Build history of the part. All positions in model axes, mm. Face numbers are marked on the shaded views. A direction names the side the tool comes from. Round coordinates to 2 decimals unless told otherwise and drop trailing zeros. Write each loop counter-clockwise with the first axis right and the second up, starting at its lowest first coordinate (ties: lowest second). Pieces come first, ordered by that corner, then holes. Notation, with made-up numbers: (43, 35.5) -> (75, 35.5) arc R20 ccw to (75, 44.5) -> close; hole circle Ø6 at (80, 44.25). An arc over 180 degrees is marked (long way). Return JSON: item names as keys, results as strings.
from build123d import *

# Parameters (mm, degrees)
F0_W      = 76.2
F0_H      = 50.8
F0_R      = 12.7
F1_DEPTH  = 19.05
F2_R      = 5.08
F3_R      = 5.08
F4_R      = 5.08
F6_DEPTH  = 2.54
F7_R      = 4.7625
F8_DEPTH  = 19.05
F10_DEPTH = 50.801


with BuildPart() as f1:
    # F0 (on Top) → F1 (new body)
    with BuildSketch(Plane.XY):
        Rectangle(F0_W, F0_H)
        Circle(F0_R, mode=Mode.SUBTRACT)
    extrude(amount=F1_DEPTH)

    # F2
    f2_edges = [f1.edges().sort_by_distance(p)[0] for p in [
        (-38.1, -25.4, 9.525),
    ]]
    fillet(f2_edges, radius=F2_R)

    # F3
    f3_edges = [f1.edges().sort_by_distance(p)[0] for p in [
        (38.1, -25.4, 9.525),
        (38.1, 25.4, 9.525),
    ]]
    fillet(f3_edges, radius=F3_R)

    # F4
    f4_edges = [f1.edges().sort_by_distance(p)[0] for p in [
        (-38.1, 25.4, 9.525),
    ]]
    fillet(f4_edges, radius=F4_R)

    # F5 (on face) → F6 (cut)
    with BuildSketch(Plane.XY.offset(19.05)):
        with BuildLine():
            Line((-29.21, 25.4), (-33.02, 25.4))
            ThreePointArc((-33.02, 25.4), (-34.3348007491, 25.2269031975), (-35.56, 24.7194090512))
            Line((-35.56, 24.7194090512), (-35.56, -24.7194090512))
            ThreePointArc((-35.56, -24.7194090512), (-34.3348007491, -25.2269031975), (-33.02, -25.4))
            Line((-33.02, -25.4), (-29.21, -25.4))
            Line((-29.21, -25.4), (-29.21, 25.4))
        make_face()
        with BuildLine():
            Line((-6.35, -10.9985226281), (-6.35, -25.4))
            Line((-6.35, -25.4), (6.35, -25.4))
            Line((6.35, -25.4), (6.35, -10.9985226281))
            ThreePointArc((6.35, -10.9985226281), (0, -12.7), (-6.35, -10.9985226281))
        make_face()
        with BuildLine():
            Line((6.35, 25.4), (-6.35, 25.4))
            Line((-6.35, 25.4), (-6.35, 10.9985226281))
            ThreePointArc((-6.35, 10.9985226281), (0, 12.7), (6.35, 10.9985226281))
            Line((6.35, 10.9985226281), (6.35, 25.4))
        make_face()
    extrude(amount=-F6_DEPTH, mode=Mode.SUBTRACT)

    # F7 (on face) → F8 (join)
    with BuildSketch(Plane.YZ.offset(38.1)):
        with Locations((0, 9.525)):
            Circle(F7_R)
    extrude(amount=F8_DEPTH)

    # F9 (on face) → F10 (cut, through all)
    with BuildSketch(Plane.XZ.offset(25.4)):
        Polygon((28.702, 19.05), (16.002, 19.05), (13.0690606325, 13.97), (31.6349393675, 13.97), align=None)
    extrude(amount=-F10_DEPTH, mode=Mode.SUBTRACT)


solid = f1.part
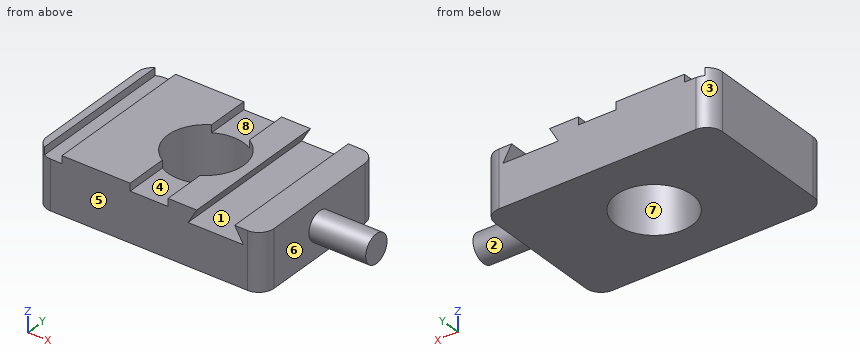
Q1. Two-plate mould, pull along X, no slides. Class the marked faces 5, 6, 7 and 8: +X half, -X half, draft (parallel to the pull), parting line (faces both ways), or undercut.
Verdict:
{"face 5": "draft", "face 6": "+X half", "face 7": "undercut", "face 8": "undercut"}
Q2. Saw through at B-B on y = 6. List the corners of the cut face in (x, z).
Verdict:
{"outline": "(-38.1, 0) -> (-11.19, 0) -> (-11.19, 19.05) -> (-29.21, 19.05) -> (-29.21, 16.51) -> (-35.56, 16.51) -> (-35.56, 19.05) -> (-38.1, 19.05) -> close; (11.19, 0) -> (38.1, 0) -> (38.1, 19.05) -> (28.7, 19.05) -> (31.63, 13.97) -> (13.07, 13.97) -> (16, 19.05) -> (11.19, 19.05) -> close"}
Q3. Saw through at A-A on x = 0. List the corners of the cut face in (y, z).
Verdict:
{"outline": "(-25.4, 0) -> (-12.7, 0) -> (-12.7, 16.51) -> (-25.4, 16.51) -> close; (12.7, 0) -> (25.4, 0) -> (25.4, 16.51) -> (12.7, 16.51) -> close"}
Q4. Saw through at C-C on z = 17.75. List the corners of the cut face in (x, y).
Verdict:
{"outline": "(-38.1, -20.32) arc R5.08 ccw to (-35.56, -24.72) -> (-35.56, 24.72) arc R5.08 ccw to (-38.1, 20.32) -> close; (-29.21, -25.4) -> (-6.35, -25.4) -> (-6.35, -11) arc R12.7 cw to (-6.35, 11) -> (-6.35, 25.4) -> (-29.21, 25.4) -> close; (6.35, -25.4) -> (15.25, -25.4) -> (15.25, 25.4) -> (6.35, 25.4) -> (6.35, 11) arc R12.7 cw to (6.35, -11) -> close; (29.45, -25.4) -> (33.02, -25.4) arc R5.08 ccw to (38.1, -20.32) -> (38.1, 20.32) arc R5.08 ccw to (33.02, 25.4) -> (29.45, 25.4) -> close"}
Q5. 3-axis set-ups, long thin cutter, end or side, ignore diameter. For the marked faces 1, 2, 3 and 4: which of +Z, -Z, +X, -X, +Y, -Y reach the whole face in a straight line?
Verdict:
{"face 1": "+Y, -Y", "face 2": "+X", "face 3": "+Z, -Z, -X, +Y", "face 4": "+Z, +Y, -Y"}
Q6. Wall check: L1, parallel to X at y = 0, z = 14; L2, parallel to X at y = 0, z = 10; L3, parallel to X at y = 9.5, z = 15.75. Give the ranges that are in metal, low to high.
Verdict:
{"L1": "x = -38.1 to -12.7, 12.7 to 13.09, 31.62 to 57.15", "L2": "x = -38.1 to -12.7, 12.7 to 57.15", "L3": "x = -38.1 to -8.43, 8.43 to 14.1, 30.61 to 38.1"}
Q7. Pin check, flat tips, straight feed: pin 1 Ø6.5 at (x, y) = (3, -16) entering from +Z; pin 2 Ø1.3 at (y, z) = (10.5, 17) entering from +X; pin 3 Ø2 at (x, z) = (38, 15) entering from +Y. Stop position of each tip, or through.
Verdict:
{"pin 1": "stops at z = 16.51", "pin 2": "stops at x = 38.1", "pin 3": "stops at y = 23.48"}
Q8. Saw through at D-D on z = 8.5. List the corners of the cut face in (x, y), then the cut area to 3 significant figures.
Verdict:
{"outline": "(-38.1, -20.32) arc R5.08 ccw to (-33.02, -25.4) -> (33.02, -25.4) arc R5.08 ccw to (38.1, -20.32) -> (38.1, -4.65) -> (57.15, -4.65) -> (57.15, 4.65) -> (38.1, 4.65) -> (38.1, 20.32) arc R5.08 ccw to (33.02, 25.4) -> (-33.02, 25.4) arc R5.08 ccw to (-38.1, 20.32) -> close; hole circle Ø25.4 at (0, 0)", "area": "3,520 mm²"}
